Design review of the part built by this model. Coordinates are the model's own, in mm. Face numbers are marked on the shaded views. A direction names the side the tool comes from. Give positions to 0.01 mm unless a question says otherwise; leave off trailing zeros. Order: outer loops, then holes, each group sorted by start corner. A loop starts at its lowest first (then second) coordinate and runs counter-clockwise, first axis right, second up. Notation, with made-up numbers: (3, 89.5) -> (25, 89.5) arc R14 cw to (25, 94.5) -> close; hole circle Ø8 at (31, 44.25). An arc over 180 degrees is marked (long way). One line per item, written item: value. Start each with the question number.
1) Tool access review of the marked faces 1, 2, 3, 4 and 5: name each direction out of +Z, -Z, +X, -X, +Y, -Y from which nothing blocks a thin tool from reaching the whole face with its end or side.
2) Consider section D-D (x = -46). State the section outline as (y, z) points.
3) Wall thickness on line 1 along Z through (x, y) = (-41.75, 73.5); line 2 along Y through (x, z) = (-53.5, 9.5); line 3 along Y through (x, z) = (-54.75, 4.75): over which ranges is each line inside the solid? List them lowest first. Write a range as from..to.
4) For pin 1 (1.5 mm diameter, centred on x = -51.5, y = 71, fed in from -Z); pin 2 (3.5 mm diameter, centred on y = 84.5, z = 1.5, fed in from -X); pin 3 (1.4 mm diameter, centred on y = 67.5, z = 9.5, fed in from +X); pin 4 (1.1 mm diameter, centred on y = 92.5, z = 1.5, fed in from -X), all flat-tipped, find the tip position at first contact; note any pin that passes through.
5) Consider section C-C (x = -54.5). State the section outline as (y, z) points.
6) Consider section A-A (y = 75). State the section outline as (x, z) points.
7) The part is to be moulded in two halves that separate along X. For the marked faces 6, 7 and 8, say which applies: released by +X, released by -X, zero draft, split by the parting line, or undercut.
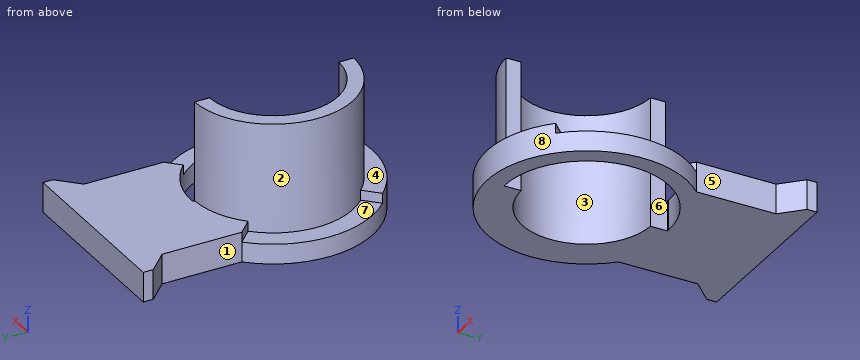
from build123d import *

# Parameters (mm, degrees)
SKETCH020_R     = 10
PAD007_DEPTH    = 3
POCKET012_DEPTH = 1
SKETCH022_R     = 8
POCKET013_DEPTH = 5
PAD008_DEPTH    = 13
POCKET014_DEPTH = 20
PAD009_DEPTH    = 3


with BuildPart() as part:
    # Sketch020 → Pad007 (new body)
    with BuildSketch(Plane.XY):
        Circle(SKETCH020_R)
    extrude(amount=PAD007_DEPTH)

    # Sketch021 (on Face3 of Pad007) → Pocket012 (cut)
    with BuildSketch(Plane.XY.offset(3)):
        with BuildLine():
            Line((0, 0), (7.071068, 7.071068))
            ThreePointArc((7.071068, -7.071068), (10, 0), (7.071068, 7.071068))
            Line((0, 0), (7.071068, -7.071068))
        make_face()
        with BuildLine():
            ThreePointArc((-7.071068, 7.071068), (-10, 0), (-7.071068, -7.071068))
            Line((0, 0), (-7.071068, -7.071068))
            Line((0, 0), (-7.071068, 7.071068))
        make_face()
    extrude(amount=-POCKET012_DEPTH, mode=Mode.SUBTRACT)

    # Sketch022 (on Face9 of Pocket012) → Pocket013 (cut)
    with BuildSketch(Plane.XY.offset(3)):
        Circle(SKETCH022_R)
    extrude(amount=-POCKET013_DEPTH, mode=Mode.SUBTRACT)

    # Sketch023 → Pad008 (join)
    with BuildSketch(Plane.XY):
        with BuildLine():
            Line((0, 6.5), (0, 8))
            ThreePointArc((0, 8), (-8, 0), (0, -8))
            Line((0, -6.5), (0, -8))
            ThreePointArc((0, 6.5), (-6.5, 0), (0, -6.5))
        make_face()
    extrude(amount=PAD008_DEPTH)

    # Sketch024 (on Face14 of Pad008) → Pocket014 (cut)
    with BuildSketch(Plane.XY.offset(13)):
        with BuildLine():
            ThreePointArc((0, -8.2), (8.2, 0), (0, 8.2))
            Line((0, 8.2), (-0.2, 8.2))
            Line((-0.2, -8.2), (-0.2, 8.2))
            Line((0, -8.2), (-0.2, -8.2))
        make_face()
    extrude(amount=-POCKET014_DEPTH, mode=Mode.SUBTRACT)

    # Sketch025 → Pad009 (join)
    with BuildSketch(Plane.XY):
        with BuildLine():
            Line((-7.071068, 7.071068), (-7.071068, 15.071068))
            Line((-7.071068, 15.071068), (-9.071068, 17.071068))
            Line((-9.071068, 18.071068), (-9.071068, 17.071068))
            Line((-9.071068, 18.071068), (9.071068, 18.071068))
            Line((9.071068, 18.071068), (9.071068, 17.071068))
            Line((9.071068, 17.071068), (7.071068, 15.071068))
            Line((7.071068, 7.071068), (7.071068, 15.071068))
            ThreePointArc((7.071068, 7.071068), (0, 10), (-7.071068, 7.071068))
        make_face()
    extrude(amount=PAD009_DEPTH)


with BuildPart() as part_1:
    # Body007 placement: moved
    add(part.part.moved(Location((-50, 75, 0))))


solid = part_1.part
Checked values:
1. face 1: +Z, -Z, -X
1. face 2: +Z, -X
1. face 3: +Z, -Z
1. face 4: +Z, -Y
1. face 5: +Z, -Z, +X
2. outline: (65.83, 0) -> (67.84, 0) -> (67.84, 3) -> (65.83, 3) -> close; (82.16, 0) -> (93.07, 0) -> (93.07, 3) -> (82.16, 3) -> close
3. line 1: z = 0..2
3. line 2: y = 67.81..69.52, 80.48..82.19
3. line 3: y = 68.56..70.56, 79.44..81.44
4. pin 1: passes through
4. pin 2: stops at x = -57.07
4. pin 3: stops at x = -50.2
4. pin 4: stops at x = -59.07
5. outline: (66.07, 0) -> (70.31, 0) -> (70.31, 13) -> (68.39, 13) -> (68.39, 3) -> (66.07, 3) -> close; (79.69, 0) -> (93.07, 0) -> (93.07, 3) -> (81.61, 3) -> (81.61, 13) -> (79.69, 13) -> close
6. outline: (-60, 0) -> (-56.5, 0) -> (-56.5, 13) -> (-58, 13) -> (-58, 2) -> (-60, 2) -> close; (-41.8, 0) -> (-40, 0) -> (-40, 2) -> (-41.8, 2) -> close
7. face 6: undercut
7. face 7: zero draft
7. face 8: split by the parting line
